Geometry: final body of the model. Coordinates: model frame, mm. A direction names the side the tool comes from. Coordinates: 2 decimals unless noted, no trailing zeros. Loops run counter-clockwise (first coordinate to the right, second up) from the corner with the lowest first, then second, coordinate; pieces in that order, holes last. Notation, with made-up numbers: (-19.5, 0.5) - (31.5, 0.5) arc R18 ccw to (31.5, 32.5) - close; hole circle Ø1 at (62.25, 45). An arc over 180 degrees is marked (long way). Answer in a Markdown table with one row per item.
from build123d import *

# Parameters (mm, degrees)
BOSS_EXTRUDE1_DEPTH = 66
SKETCH2_R           = 8.5
BOSS_EXTRUDE2_DEPTH = 8
CHAMFER1_SIZE       = 4


with BuildPart() as part:
    # Sketch1 → Boss-Extrude1 (new body)
    with BuildSketch(Plane.XY):
        with BuildLine():
            Line((3.122498999, 9.5), (13.377501001, 9.5))
            ThreePointArc((13.377501001, 9.5), (26.5, 0), (13.377501001, -9.5))
            Line((13.377501001, -9.5), (3.122498999, -9.5))
            ThreePointArc((3.122498999, -9.5), (-10, 0), (3.122498999, 9.5))
        make_face()
    extrude(amount=BOSS_EXTRUDE1_DEPTH)

    # Sketch2 → Boss-Extrude2 (add)
    with BuildSketch(Plane.XY.offset(66)):
        with Locations((8.25, 0)):
            Circle(SKETCH2_R)
    extrude(amount=BOSS_EXTRUDE2_DEPTH)

    # Chamfer1
    chamfer1_edges = [part.edges().sort_by_distance(p)[0] for p in [
        (-0.25, 0, 74),
    ]]
    chamfer(chamfer1_edges, length=CHAMFER1_SIZE)


solid = part.part
(1) First-contact query: pin 1 Ø8 at (y, z) = (0.5, 56) entering from +X; pin 2 Ø3 at (x, z) = (9, 47) entering from +Y; pin 3 Ø4 at (x, y) = (21, 0.5) entering from +Z; pin 4 Ø11.5 at (x, z) = (8.5, 29.5) entering from +Y. Flat tips, straight axial feed; report the tip coordinate or a pass-through.
Verdict:
| item | result |
|---|---|
| pin 1 | stops at x = 26.5 |
| pin 2 | stops at y = 9.5 |
| pin 3 | stops at z = 66 |
| pin 4 | stops at y = 9.74 |
(2) Ray query, probe 1 along Y at (x, z) = (11, 22); probe 2 along Z at (x, y) = (24.5, -4.75); probe 3 along Y at (x, z) = (16.5, 52.5). Return the intervals inside material, ascending.
Verdict:
| item | result |
|---|---|
| probe 1 | y = -9.5 to 9.5 |
| probe 2 | z = 0 to 66 |
| probe 3 | y = -10 to 10 |
(3) Cut plane A-A on x = 8.25. Output: boundary loops of the cut face in (y, z), then the cut area to 3 significant figures.
Verdict:
| item | result |
|---|---|
| outline | (-9.5, 0) - (9.5, 0) - (9.5, 66) - (8.5, 66) - (8.5, 70) - (4.5, 74) - (-4.5, 74) - (-8.5, 70) - (-8.5, 66) - (-9.5, 66) - close |
| area | 1,370 mm² |
(4) Access query for faces 4 (the face through (26.497, 0.264, 32.538)), 5 (the face through (8, 9.5, 33)), 6 (the face through (17, 2, 66)). Directions: +Z, -Z, +X, -X, +Y, -Y. A direction counts if a zero-diameter tool reaches every point of the face in a straight line with its end or side. Return the directions, or none.
Verdict:
| item | result |
|---|---|
| face 4 | +Z, -Z |
| face 5 | +Z, -Z, +Y |
| face 6 | +Z |
(5) Cut plane B-B on z = 33. Output: boundary loops of the cut face in (x, y), then the cut area to 3 significant figures.
Verdict:
| item | result |
|---|---|
| outline | (3.12, -9.5) - (13.38, -9.5) arc R10 ccw (long way) to (13.38, 9.5) - (3.12, 9.5) arc R10 ccw (long way) to start |
| area | 632 mm² |
(6) Pull-direction query (X, two-part tool) for faces 1 (the face through (8, -9.5, 33)), 2 (the face through (9, 0, 0)), 3 (the face through (1.985, 5.745, 67.972)); classes: pulls with the +X half, pulls with the -X half, needs draft (parallel to the pull), parting line crosses it, or undercut.
Verdict:
| item | result |
|---|---|
| face 1 | undercut |
| face 2 | needs draft |
| face 3 | parting line crosses it |
